from build123d import *

# Parameters (mm, degrees)
SKETCH1_W                                         = 48.006
SKETCH1_H                                         = 28.575
BOSS_EXTRUDE1_DEPTH                               = 3.175
CSK_FOR_6_FLAT_HEAD_MACHINE_SCREW_100_D           = 3.7973
CSK_FOR_6_FLAT_HEAD_MACHINE_SCREW_100_CSINK_D     = 7.0866
CSK_FOR_6_FLAT_HEAD_MACHINE_SCREW_100_CSINK_ANGLE = 100
LPATTERN1_COUNT                                   = 2
LPATTERN1_PITCH                                   = 12.7
LPATTERN1_COL_COUNT                               = 2
LPATTERN1_COL_PITCH                               = 12.7


with BuildPart() as part:
    # Sketch1 → Boss-Extrude1 (new body)
    with BuildSketch(Plane(origin=(0, 0, 0), x_dir=(1, 0, 0), z_dir=(0, 1, 0))):
        with Locations((-24.003, 14.2875)):
            Rectangle(SKETCH1_W, SKETCH1_H)
    extrude(amount=BOSS_EXTRUDE1_DEPTH)

    # CSK for #6 Flat Head Machine Screw (100)1 (through all)
    with Locations(Plane(origin=(0, 3.175, 0), x_dir=(1, 0, 0), z_dir=(0, 1, 0))):
        with Locations((-24.003, 15.875)):
            csk_for_6_flat_head_machine_screw_100 = CounterSinkHole(CSK_FOR_6_FLAT_HEAD_MACHINE_SCREW_100_D / 2, CSK_FOR_6_FLAT_HEAD_MACHINE_SCREW_100_CSINK_D / 2, counter_sink_angle=CSK_FOR_6_FLAT_HEAD_MACHINE_SCREW_100_CSINK_ANGLE)

    # LPattern1: CSK for #6 Flat Head Machine Screw (100)1 ×2
    with Locations(*[(i * LPATTERN1_PITCH, 0, 0) for i in range(1, LPATTERN1_COUNT)]):
        add(csk_for_6_flat_head_machine_screw_100, mode=Mode.SUBTRACT)

    # LPattern1 col: CSK for #6 Flat Head Machine Screw (100)1 ×2
    with Locations(*[(-i * LPATTERN1_COL_PITCH, 0, 0) for i in range(1, LPATTERN1_COL_COUNT)]):
        add(csk_for_6_flat_head_machine_screw_100, mode=Mode.SUBTRACT)


solid = part.part
Work out the finished part from the listing and answer in its coordinate system (mm). Give positions to 0.01 mm unless a question says otherwise; leave off trailing zeros. Write each loop counter-clockwise with the first axis right and the second up, starting at its lowest first coordinate (ties: lowest second). Pieces come first, ordered by that corner, then holes. Notation, with made-up numbers: (-32, 37) - (25, 37) arc R17 ccw to (25, 42) - close; hole circle Ø8 at (19.5, 75). An arc over 180 degrees is marked (long way). One line per item, written item: value. Start each with the question number.
1. For a pull along Z with two mould halves and no side action, classify faces 1 (the flat face through (-24, 2, -28.575)), 2 (the flat face through (-24, 3.175, -11)), 3 (the cylindrical face through (-22.604, 0.885, -17.158)), 4 (the flat face through (-24, 2, 0)) as +Z half, -Z half, draft (parallel to the pull), parting line (faces both ways), or undercut.
2. Consider probe 1 along X at (y, z) = (0.1, -14.5); probe 2 along X at (y, z) = (1.35, -17); probe 3 along Z at (x, y) = (-23, 2.4) (3 decimals). Determine where each line is inside the solid, lowest interval first.
3. Find section A-A (y = 2.3). Write down the section's boundary in (x, z) (3 decimals), then the cut area to 3 significant figures.
4. Given pin 1 (6 mm diameter, centred on x = -11.303, z = -15.875, fed in from +Y), flat-ended and moving along its own axis, determine where the tip first touches the part or whether it passes through.
5. Find section B-B (z = -17.25). State how many separate pieces and enclosed holes the cut face has, then the cut area to 3 significant figures.
Geometry results:
1. face 1: -Z half
1. face 2: draft
1. face 3: undercut
1. face 4: +Z half
2. probe 1: -48.01 to -38.01, -35.39 to -25.31, -22.69 to -12.61, -9.99 to 0
2. probe 2: -48.01 to -38.23, -35.17 to -25.53, -22.47 to -12.83, -9.77 to 0
2. probe 3: -28.575 to -18.295, -13.455 to 0
3. outline: (-48.006, -28.575) - (0, -28.575) - (0, 0) - (-48.006, 0) - close; hole circle Ø5.001 at (-36.703, -15.875); hole circle Ø5.001 at (-24.003, -15.875); hole circle Ø5.001 at (-11.303, -15.875)
3. area: 1,310 mm2
4. pin 1: y = 2.72
5. separate pieces: 4
5. enclosed holes: 0
5. area: 119 mm2
